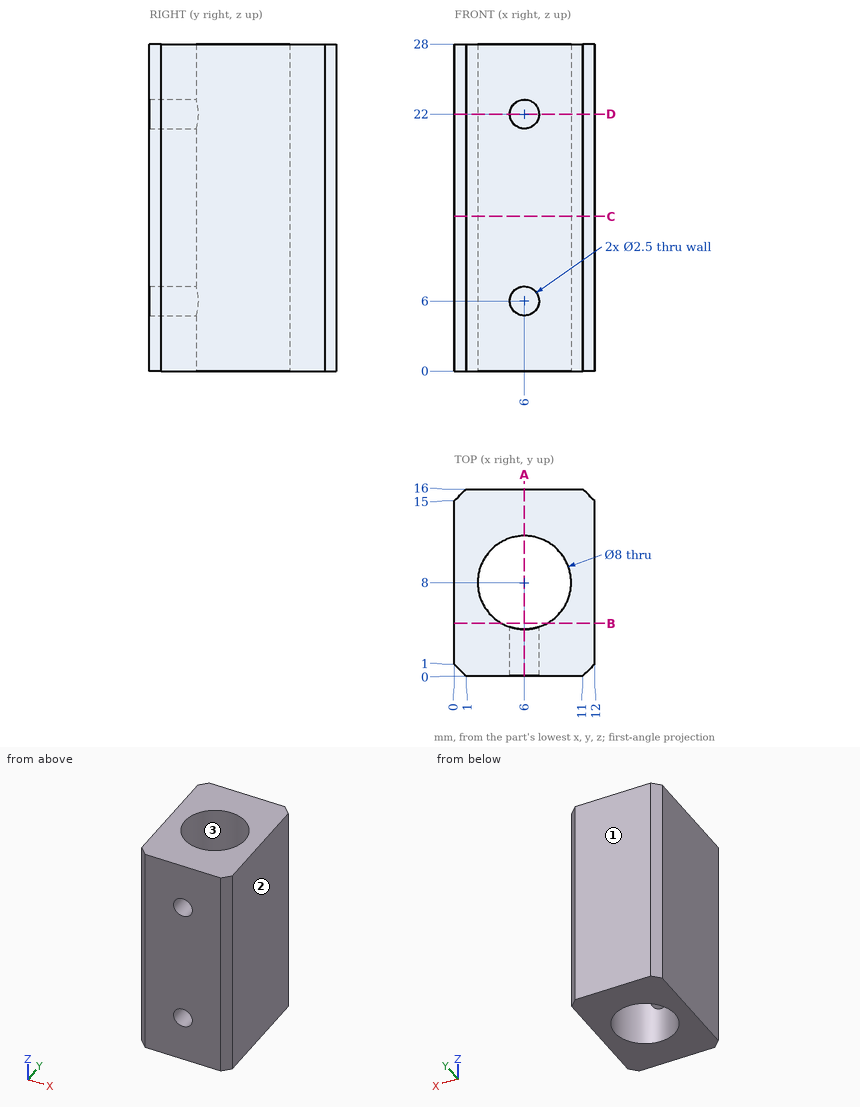
Verification items for this drawing (mm, ordinates from the low corner). Coordinates: 2 decimals unless noted, no trailing zeros. Write each loop counter-clockwise with the first axis right and the second up, starting at its lowest first coordinate (ties: lowest second). Pieces come first, ordered by that corner, then holes. Notation, with made-up numbers: (63.25, -18) -> (118.25, -18) arc R14 ccw to (118.25, 0) -> close; hole circle Ø5 at (73, 49.5). An arc over 180 degrees is marked (long way). One line per item, written item: value. Start each with the question number.
Q1. Cross-section at D-D on z = 22. Enter the section's corners in (x, y).
Q2. Cross-section at A-A on x = 6. Enter the section's corners in (y, z).
Q3. Cross-section at C-C on z = 13.25. Enter the section's corners in (x, y), and give its area (3 significant figures).
Q4. Thickness scan on L1, parallel to Z at x = 6, y = 3.1; L2, parallel to Y at x = 6, z = 9.5; L3, parallel to X at y = 9.75, z = 25. Record the ranges inside material, lowest first. Write a range as from..to.
Q5. Go/stop test with a flat-tipped pin: P1, Ø7, axis at x = 6, y = 8, coming from the -Z side. Record where the tip stops, or that it passes through.
Q6. Mould release check, pull along Y, two halves, no side actions. Record for the marked faces 1, 2 and 3: pulls with the +Y half, pulls with the -Y half, needs draft (parallel to the pull), parting line crosses it, or undercut.
Q7. Cross-section at B-B on y = 4.5. Enter the section's corners in (x, z), and give its area (3 significant figures).
Checked values:
1. outline: (0, 1) -> (1, 0) -> (4.75, 0) -> (4.75, 4.2) arc R4 cw (long way) to (7.25, 4.2) -> (7.25, 0) -> (11, 0) -> (12, 1) -> (12, 15) -> (11, 16) -> (1, 16) -> (0, 15) -> close
2. outline: (0, 0) -> (4, 0) -> (4, 4.75) -> (0, 4.75) -> close; (0, 7.25) -> (4, 7.25) -> (4, 20.75) -> (0, 20.75) -> close; (0, 23.25) -> (4, 23.25) -> (4, 28) -> (0, 28) -> close; (12, 0) -> (16, 0) -> (16, 28) -> (12, 28) -> close
3. outline: (0, 1) -> (1, 0) -> (11, 0) -> (12, 1) -> (12, 15) -> (11, 16) -> (1, 16) -> (0, 15) -> close; hole circle Ø8 at (6, 8)
3. area: 140 mm²
4. L1: z = 0..4.75, 7.25..20.75, 23.25..28
4. L2: y = 0..4, 12..16
4. L3: x = 0..2.4, 9.6..12
5. P1: passes through
6. face 1: pulls with the +Y half
6. face 2: needs draft
6. face 3: undercut
7. outline: (0, 0) -> (4.06, 0) -> (4.06, 28) -> (0, 28) -> close; (7.94, 0) -> (12, 0) -> (12, 28) -> (7.94, 28) -> close
7. area: 228 mm²
